```python
from build123d import *

# Parameters (mm, degrees)
SKETCH_1_R                   = 7.5
EXTRUDE_1_DEPTH              = 10
HOLE_WIZARD_M4_1_D           = 4.5
HOLE_WIZARD_M4_1_CBORE_D     = 8
HOLE_WIZARD_M4_1_CBORE_DEPTH = 4.6


with BuildPart() as part:
    # 草图1 → 凸台-拉伸1 (new body)
    with BuildSketch(Plane(origin=(0, 0, 0), x_dir=(0, 0, -1), z_dir=(1, 0, 0))):
        Polygon((0, 0), (50, 0), (50, 15), (35, 15), (35, 32), (15, 32), (15, 15), (0, 15), align=None)
        with Locations((25, 20)):
            Circle(SKETCH_1_R, mode=Mode.SUBTRACT)
    extrude(amount=EXTRUDE_1_DEPTH)

    # M4 六角圆柱头螺钉的柱形沉头孔1 (through all)
    with Locations(Plane(origin=(5, 15, -43), x_dir=(0, 0, 1), z_dir=(0, 1, 0))):
        with Locations((0, 0), (36, 0)):
            CounterBoreHole(HOLE_WIZARD_M4_1_D / 2, HOLE_WIZARD_M4_1_CBORE_D / 2, HOLE_WIZARD_M4_1_CBORE_DEPTH)


solid = part.part
```
Geometry: final body of the model. Coordinates: model frame, mm. A direction names the side the tool comes from. Coordinates: 2 decimals unless noted, no trailing zeros. Order: outer loops, then holes, each group sorted by start corner. A loop starts at its lowest first (then second) coordinate and runs counter-clockwise, first axis right, second up. Notation, with made-up numbers: (84.25, 60) - (100.25, 60) arc R26 ccw to (100.25, 96) - close; hole circle Ø11 at (24.25, 26). An arc over 180 degrees is marked (long way). Return JSON: item names as keys, results as strings. Group by question number.
1. Material intervals for line 1 along X through (y, z) = (14.1, -7); line 2 along X through (y, z) = (4, -43); line 3 along Y through (x, z) = (7, -25), sorted ascending. Write a range as [from, to].
2. Cut plane D-D (y = 5). Output: boundary loops of the cut face in (x, z).
3. Pin query (flat end, axial travel): pin 1 (5 mm diameter, centred on x = 6.5, y = 23, fed in from +Z); pin 2 (6 mm diameter, centred on x = 5, z = -7, fed in from +Y); pin 3 (3 mm diameter, centred on x = 3.5, z = -40, fed in from +Y). Return the tip coordinate at first contact, or that it passes through.
4. Set-up query: faces 5 (the face through (3, 15, -39)), 6 (the face through (3, 15, -11)), 7 (the face through (5, 8, 0)), 8 (the face through (3, 10.4, -5)), 9 (the face through (5, 32, -25)). Return all of +Z, -Z, +X, -X, +Y, -Y with unobstructed straight access to the full face (end or side cutting, diameter ignored); none if empty.
5. Pull-direction query (X, two-part tool) for faces 1 (the face through (0, 9, -25)), 2 (the face through (5.099, 5.127, -40.752)), 3 (the face through (5, 7, -50)), 4 (the face through (1.095, 12.732, -7.867)); classes: pulls with the +X half, pulls with the -X half, needs draft (parallel to the pull), parting line crosses it, or undercut.
6. Cut plane C-C (y = 20). Output: boundary loops of the cut face in (x, z), plus the area to 3 significant figures.
7. Cut plane A-A (x = 5). Output: boundary loops of the cut face in (y, z).
8. Cut plane B-B (z = -25). Output: boundary loops of the cut face in (x, y), plus the area to 3 significant figures.
Resolved:
{
 "1": {"line 1": "x = [0, 1], [9, 10]", "line 2": "x = [0, 2.75], [7.25, 10]", "line 3": "y = [0, 12.5], [27.5, 32]"},
 "2": {"outline": "(0, -50) - (10, -50) - (10, 0) - (0, 0) - close; hole circle Ø4.5 at (5, -43); hole circle Ø4.5 at (5, -7)"},
 "3": {"pin 1": "stops at z = -15", "pin 2": "stops at y = 10.4", "pin 3": "stops at y = 15"},
 "4": {"face 5": "-Z, +X, -X, +Y", "face 6": "+Z, +X, -X, +Y", "face 7": "+Z, +X, -X, +Y, -Y", "face 8": "+Y", "face 9": "+Z, -Z, +X, -X, +Y"},
 "5": {"face 1": "pulls with the -X half", "face 2": "undercut", "face 3": "needs draft", "face 4": "undercut"},
 "6": {"outline": "(0, -35) - (10, -35) - (10, -32.5) - (0, -32.5) - close; (0, -17.5) - (10, -17.5) - (10, -15) - (0, -15) - close", "area": "50.0 mm²"},
 "7": {"outline": "(0, -50) - (15, -50) - (15, -47) - (10.4, -47) - (10.4, -45.25) - (0, -45.25) - close; (0, -40.75) - (10.4, -40.75) - (10.4, -39) - (15, -39) - (15, -35) - (32, -35) - (32, -15) - (15, -15) - (15, -11) - (10.4, -11) - (10.4, -9.25) - (0, -9.25) - close; (0, -4.75) - (10.4, -4.75) - (10.4, -3) - (15, -3) - (15, 0) - (0, 0) - close; hole circle Ø15 at (20, -25)"},
 "8": {"outline": "(0, 0) - (10, 0) - (10, 12.5) - (0, 12.5) - close; (0, 27.5) - (10, 27.5) - (10, 32) - (0, 32) - close", "area": "170 mm²"}
}
